Check sheet for the modelled part. Datum: model origin and axes. Units: mm. Face numbers are marked on the shaded views. Coordinates: 2 decimals unless noted, no trailing zeros. Order: outer loops, then holes, each group sorted by start corner. A loop starts at its lowest first (then second) coordinate and runs counter-clockwise, first axis right, second up.
1. Cross-section at C-C (z = -25). Enter the section's corners in (x, y) (3 decimals).
2. Cross-section at A-A (x = 1.5). Enter the section's corners in (y, z).
3. Cross-section at D-D (z = -17.5). Enter the section's corners in (x, y).
4. Cross-section at B-B (x = -25). Enter the section's corners in (y, z) (3 decimals), then the cut area to 3 significant figures.
5. Thickness scan on line 1 (Z direction, x = -25, y = 1.5) (3 decimals); line 2 (X direction, y = 5, z = 25) (3 decimals); line 3 (X direction, y = 2, z = 17.5). Record the ranges inside material, lowest first.
6. Draft check along X on the marked faces 1, 2 and 3. Enter one of: released by +X, released by -X, zero draft, split by the parting line, or undercut.
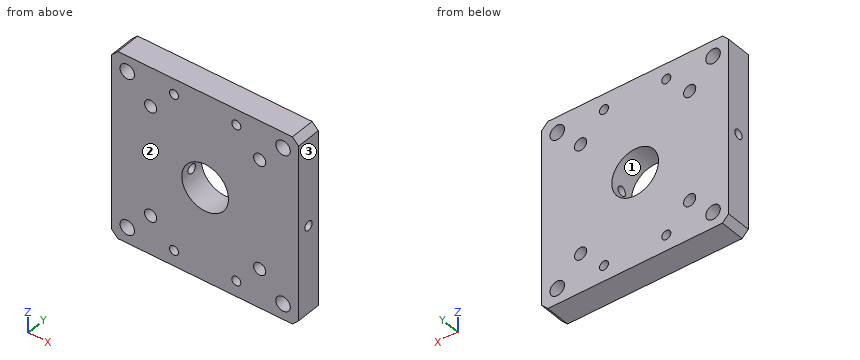
Autodesk Inventor part; units mm, degrees
ref_plane "YZ Plane" through (0, 0, 0) normal (1, 0, 0) x (0, 1, 0)
ref_plane "XZ Plane" through (0, 0, 0) normal (0, 1, 0) x (-1, 0, 0)
ref_plane "XY Plane" through (0, 0, 0) normal (0, 0, 1) x (1, 0, 0)
sketch "Sketch1" plane through (0, 0, 0) normal (0, 1, 0) x (-1, 0, 0)
  line L0 (-30, -30) -> (30, -30)
  line L1 (30, -30) -> (30, 30)
  line L2 (30, 30) -> (-30, 30)
  line L3 (-30, 30) -> (-30, -30)
  line L4 (-30, -30) -> (30, 30) construction
  line L5 (30, -30) -> (-30, 30) construction
  circle A0 centre (0, 0) radius 7.5
  circle A1 centre (-25, 25) radius 1.95
  circle A2 centre (0, 25) radius 1.95
  circle A3 centre (0, 25) radius 1.95
  circle A4 centre (25, 0) radius 1.95
  circle A5 centre (25, -25) radius 1.95
  circle A6 centre (-25, 25) radius 1.95
  circle A7 centre (-25, -25) radius 1.95
  circle A8 centre (25, 25) radius 1.95
  circle A9 centre (-25, 0) radius 1.95
  circle A10 centre (0, -25) radius 1.95
  line L6 (28, 30) -> (30, 28)
  line L7 (30, 28) -> (30, -28)
  line L8 (30, -28) -> (28, -30)
  line L9 (28, -30) -> (-28, -30)
  line L10 (-28, -30) -> (-30, -28)
  line L11 (-30, -28) -> (-30, 28)
  line L12 (-30, 28) -> (-28, 30)
  line L13 (-28, 30) -> (28, 30)
  dimension "d0" = 60
  dimension "d1" = 60
  dimension "d13" = 15
extrude "Extrusion1" add sketch "Sketch1" along normal blind 8 contours L3 L10 L0 | L10 L3 L12 L2 L6 L1 L8 L0 | L8 L1 L0 | L3 L2 L12 | L6 L2 L1 | A1 | A2 | A4 | A5 | A7 | A8 | A9 | A10
sketch "Sketch2" plane through (0, 8, 0) normal (0, 1, 0) x (1, 0, 0)
  line L0 (30, 30) -> (-30, 30)
  line L1 (-30, 30) -> (-30, -30)
  line L2 (-30, -30) -> (30, -30)
  line L3 (30, -30) -> (30, 30)
  line L4 (17.5, -17.5) -> (-17.5, -17.5)
  line L5 (-17.5, -17.5) -> (-17.5, 17.5)
  line L6 (-17.5, 17.5) -> (17.5, 17.5)
  line L7 (17.5, 17.5) -> (17.5, -17.5)
  line L8 (17.5, -17.5) -> (-17.5, 17.5) construction
  line L9 (-17.5, -17.5) -> (17.5, 17.5) construction
  line L10 (0, -17.5) -> (0, 17.5)
  line L11 (-17.5, 0) -> (17.5, 0)
  point P0 (0, 0)
  dimension "d4" = 35
  dimension "d5" = 35
hole "Hole1" at (-17.5, 8, 17.5) at (-17.5, 8, -17.5) at (17.5, 8, -17.5) at (17.5, 8, 17.5) direction (0, -1, 0) diameter 3.9 depth 10 tip angle 118
chamfer "Chamfer1" distance 2 angle 45 4 edges at (30, 4, 30) (30, 4, -30) (-30, 4, -30) (-30, 4, 30)
sketch "Sketch3" plane through (0, 8, 0) normal (0, 1, 0) x (1, 0, 0)
  line L0 (-28, -30) -> (-30, -28)
  line L1 (-28, -30) -> (28, -30)
  line L2 (30, -28) -> (28, -30)
  line L3 (30, -28) -> (30, 28)
  line L4 (28, 30) -> (30, 28)
  line L5 (28, 30) -> (-28, 30)
  line L6 (-30, 28) -> (-28, 30)
  line L7 (-30, 28) -> (-30, -28)
  circle A0 centre (17.5, 17.5) radius 1.95
  circle A1 centre (-17.5, -17.5) radius 1.95
  circle A2 centre (-17.5, 17.5) radius 1.95
  circle A3 centre (17.5, -17.5) radius 1.95
  circle A4 centre (0, 0) radius 7.5
  line L8 (25, -25) -> (-25, -25)
  line L9 (-25, -25) -> (-25, 25)
  line L10 (-25, 25) -> (25, 25)
  line L11 (25, 25) -> (25, -25)
  line L12 (25, -25) -> (-25, 25) construction
  line L13 (-25, -25) -> (25, 25) construction
  dimension "d17" = 50
  dimension "d18" = 50
hole "Hole2" at (-25, 8, -25) at (25, 8, -25) at (25, 8, 25) at (-25, 8, 25) direction (0, -1, 0) diameter 4.65 end through all
sketch "Sketch4" plane through (30, 0, 28) normal (1, 0, 0) x (0, 0, -1)
  line L0 (56, 8) -> (56, 0)
  line L1 (0, 8) -> (56, 8)
  line L2 (0, 0) -> (0, 8)
  line L3 (0, 0) -> (56, 0)
  circle A0 centre (28, 4) radius 1.5
  line L4 (-2, 8) -> (-2, 0)
  point P0 (28, 0)
  dimension "d26" = 3
  dimension "d27" = 4
  dimension "d28" = 30
extrude "Extrusion2" cut sketch "Sketch4" against normal through all contours A0
sketch "Sketch5" plane through (0, 8, 0) normal (0, 1, 0) x (1, 0, 0)
  circle A0 centre (25, -25) radius 2.325
  circle A1 centre (-25, -25) radius 2.325
  circle A2 centre (25, 25) radius 2.325
  circle A3 centre (-25, 25) radius 2.325
  circle A4 centre (10, -25) radius 1.45
  circle A5 centre (-10, -25) radius 1.45
  circle A6 centre (10, 25) radius 1.45
  circle A7 centre (-10, 25) radius 1.45
  point P0 (0, 0)
  dimension "d31" = 2.9
  dimension "d32" = 2.9
  dimension "d33" = 15
  dimension "d34" = 15
  dimension "d35" = 2.9
  dimension "d36" = 2.9
extrude "Extrusion3" cut sketch "Sketch5" against normal blind 10 contours A4 | A5 | A6 | A7
properties part number "00_XY_stage-CHUO_SEIKI_LD-647-R1-Top"
Data:
1. outline: (-30, 0) - (-27.325, 0) - (-27.325, 8) - (-30, 8) - close; (-22.675, 0) - (-11.45, 0) - (-11.45, 8) - (-22.675, 8) - close; (-8.55, 0) - (8.55, 0) - (8.55, 8) - (-8.55, 8) - close; (11.45, 0) - (22.675, 0) - (22.675, 8) - (11.45, 8) - close; (27.325, 0) - (30, 0) - (30, 8) - (27.325, 8) - close
2. outline: (0, -30) - (8, -30) - (8, -7.35) - (0, -7.35) - close; (0, 7.35) - (8, 7.35) - (8, 30) - (0, 30) - close
3. outline: (-30, 0) - (-19.45, 0) - (-19.45, 8) - (-30, 8) - close; (-15.55, 0) - (15.55, 0) - (15.55, 8) - (-15.55, 8) - close; (19.45, 0) - (30, 0) - (30, 8) - (19.45, 8) - close
4. outline: (0, -30) - (8, -30) - (8, -27.325) - (0, -27.325) - close; (0, -22.675) - (8, -22.675) - (8, 22.675) - (0, 22.675) - close; (0, 27.325) - (8, 27.325) - (8, 30) - (0, 30) - close; hole circle Ø3 at (4, 0)
4. area: 399 mm2
5. line 1: z = -30 to -27.325, -22.675 to 22.675, 27.325 to 30
5. line 2: x = -30 to -27.325, -22.675 to -11.45, -8.55 to 8.55, 11.45 to 22.675, 27.325 to 30
5. line 3: x = -30 to -19.45, -15.55 to 15.55, 19.45 to 30
6. face 1: undercut
6. face 2: zero draft
6. face 3: released by +X
